Geometry check sheet. Reference: drawing and pictorial views, mm from the part's lowest x, y, z. Round coordinates to 2 decimals unless told otherwise and drop trailing zeros. Write each loop counter-clockwise with the first axis right and the second up, starting at its lowest first coordinate (ties: lowest second). Pieces come first, ordered by that corner, then holes. Notation, with made-up numbers: (-30.75, 52.5) -> (-20.75, 52.5) arc R14 ccw to (-20.75, 61.5) -> close; hole circle Ø1 at (7.5, -9). An arc over 180 degrees is marked (long way). Answer as a JSON object with one key per item and string values. Group by question number.
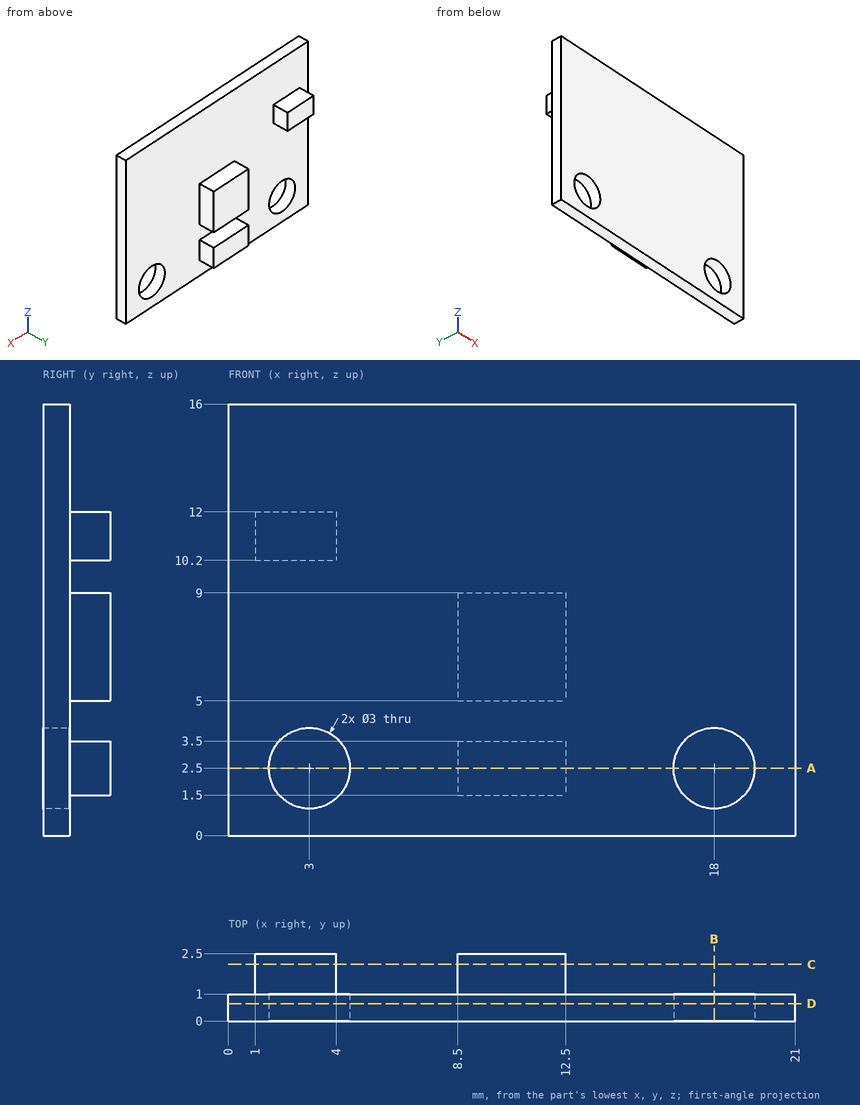
(1) Section check C-C on y = 2.1. Record the cut outline in (x, z).
(2) Section check D-D on y = 0.65. Record the cut outline in (x, z).
(3) Scan lines: line 1 along X through (y, z) = (0.6, 2.5); line 2 along Z through (x, y) = (17.25, 0.45); line 3 along Y through (x, z) = (5.75, 10.5). Record each from-to range of solid material in increasing order.
(4) Go/stop test with flat-tipped pins: pin 1 Ø1.2 at (y, z) = (2, 7) entering from +X; pin 2 Ø0.8 at (x, y) = (11, 2) entering from +Z; pin 3 Ø5 at (x, z) = (19, 10.5) entering from +Y; pin 4 Ø4 at (x, z) = (3, 2.5) entering from -Y. Record where each tip stops, or that it passes through.
(5) Section check A-A on z = 2.5. Record the cut outline in (x, y).
(6) Section check B-B on x = 18. Record the cut outline in (y, z), then the cut area to 3 significant figures.
Data:
{
 "1": {"outline": "(1, 10.2) -> (4, 10.2) -> (4, 12) -> (1, 12) -> close; (8.5, 1.5) -> (12.5, 1.5) -> (12.5, 3.5) -> (8.5, 3.5) -> close; (8.5, 5) -> (12.5, 5) -> (12.5, 9) -> (8.5, 9) -> close"},
 "2": {"outline": "(0, 0) -> (21, 0) -> (21, 16) -> (0, 16) -> close; hole circle Ø3 at (3, 2.5); hole circle Ø3 at (18, 2.5)"},
 "3": {"line 1": "x = 0 to 1.5, 4.5 to 16.5, 19.5 to 21", "line 2": "z = 0 to 1.2, 3.8 to 16", "line 3": "y = 0 to 1"},
 "4": {"pin 1": "stops at x = 12.5", "pin 2": "stops at z = 9", "pin 3": "stops at y = 1", "pin 4": "stops at y = 0"},
 "5": {"outline": "(0, 0) -> (1.5, 0) -> (1.5, 1) -> (0, 1) -> close; (4.5, 0) -> (16.5, 0) -> (16.5, 1) -> (12.5, 1) -> (12.5, 2.5) -> (8.5, 2.5) -> (8.5, 1) -> (4.5, 1) -> close; (19.5, 0) -> (21, 0) -> (21, 1) -> (19.5, 1) -> close"},
 "6": {"outline": "(0, 0) -> (1, 0) -> (1, 1) -> (0, 1) -> close; (0, 4) -> (1, 4) -> (1, 16) -> (0, 16) -> close", "area": "13.0 mm²"}
}
